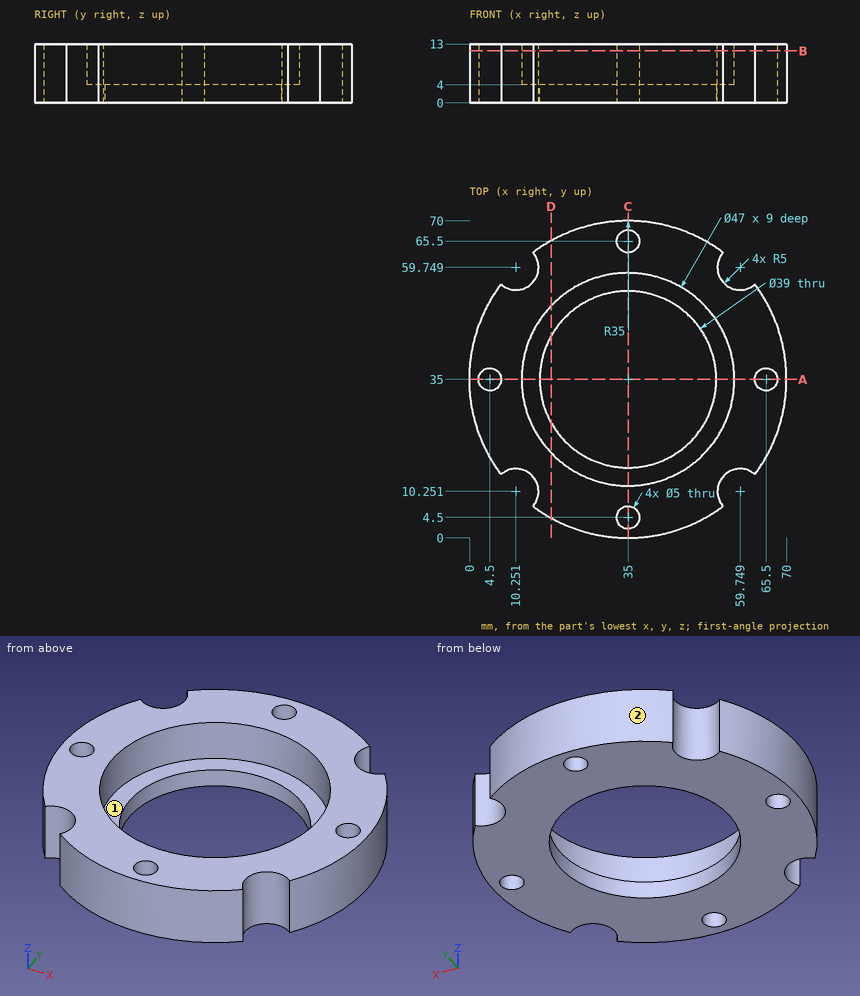
Check sheet for the drawn part. Datum: minimum x, y, z corner. Units: mm. A direction names the side the tool comes from. Give positions to 0.01 mm unless a question says otherwise; leave off trailing zeros. Order: outer loops, then holes, each group sorted by start corner. A loop starts at its lowest first (then second) coordinate and runs counter-clockwise, first axis right, second up. Notation, with made-up numbers: (-15, 23.5) - (32, 23.5) arc R12 ccw to (32, 41.5) - close; hole circle Ø7 at (31, 7.5). An arc over 180 degrees is marked (long way). Answer in a Markdown table with one row per item. Add a question column.
Q1. Cross-section at D-D, the plane x = 18. Enter the section's corners in (y, z) (1 decimal).
Q2. Cross-section at A-A, the plane y = 35. Enter the section's corners in (x, z), then the cut area to 3 significant figures.
Q3. Cross-section at B-B, the plane z = 11.5. Enter the section's corners in (x, y).
Q4. Material ranges on probe 1 along Y at (x, z) = (35, 6.5); probe 2 along Y at (x, z) = (30.5, 3.25); probe 3 along Y at (x, z) = (46.5, 4.5) (1 decimal), recorded low to high. Write a range as from..to.
Q5. Tool access check on the marked faces 1 and 2. Record the directions out of +Z, -Z, +X, -X, +Y, -Y that give a thin tool (end or side, any length) a straight path to the whole face; none if there is none.
Q6. Gauge pin test, flat ends, axial feed: pin 1 (1.5 mm diameter, centred on y = 32, z = 5, fed in from -X); pin 2 (5 mm diameter, centred on x = 7.5, z = 1.5, fed in from -Y); pin 3 (5 mm diameter, centred on y = 30, z = 8, fed in from +X). Record the tip position at first contact, or that the pin passes through.
Check values:
| question | item | result |
|---|---|---|
| 1 | outline | (4.4, 0) - (25.4, 0) - (25.4, 4) - (18.8, 4) - (18.8, 13) - (4.4, 13) - close; (44.6, 0) - (65.6, 0) - (65.6, 13) - (51.2, 13) - (51.2, 4) - (44.6, 4) - close |
| 2 | outline | (0, 0) - (2, 0) - (2, 13) - (0, 13) - close; (7, 0) - (15.5, 0) - (15.5, 4) - (11.5, 4) - (11.5, 13) - (7, 13) - close; (54.5, 0) - (63, 0) - (63, 13) - (58.5, 13) - (58.5, 4) - (54.5, 4) - close; (68, 0) - (70, 0) - (70, 13) - (68, 13) - close |
| 2 | area | 201 mm^2 |
| 3 | outline | (6.98, 14.03) arc R5 cw to (14.03, 6.98) arc R35 ccw to (55.97, 6.98) arc R5 cw to (63.02, 14.03) arc R35 ccw to (63.02, 55.97) arc R5 cw to (55.97, 63.02) arc R35 ccw to (14.03, 63.02) arc R5 cw to (6.98, 55.97) arc R35 ccw to start; hole circle Ø5 at (4.5, 35); hole circle Ø47 at (35, 35); hole circle Ø5 at (35, 4.5); hole circle Ø5 at (35, 65.5); hole circle Ø5 at (65.5, 35) |
| 4 | probe 1 | y = 0..2, 7..11.5, 58.5..63, 68..70 |
| 4 | probe 2 | y = 0.29..16.03, 53.97..69.71 |
| 4 | probe 3 | y = 1.9..14.5, 55.5..68.1 |
| 5 | face 1 | +Z |
| 5 | face 2 | +Z, -Z, +Y |
| 6 | pin 1 | stops at x = 0.07 |
| 6 | pin 2 | stops at y = 14.03 |
| 6 | pin 3 | stops at x = 69.91 |
